Input: part model. Units: mm. Frame: model coordinates. Face numbers are marked on the shaded views. A direction names the side the tool comes from. Coordinates: 2 decimals unless noted, no trailing zeros. Write each loop counter-clockwise with the first axis right and the second up, starting at its lowest first coordinate (ties: lowest second). Pieces come first, ordered by that corner, then holes. Notation, with made-up numbers: (47.5, 44.5) -> (89.5, 44.5) arc R3 ccw to (89.5, 49.5) -> close; hole circle Ø3 at (28.25, -29). An arc over 180 degrees is marked (long way). Use one line per item in the form item = value. Start each with the question number.
(1) Set-up query: the marked faces 1 and 2. Return all of +Z, -Z, +X, -X, +Y, -Y with unobstructed straight access to the full face (end or side cutting, diameter ignored); none if empty.
(2) Pull-direction query (Z, two-part tool) for the marked faces 3, 4, 5 and 6; classes: released by +Z, released by -Z, zero draft, split by the parting line, or undercut.
(3) First-contact query: pin 1 (2.5 mm diameter, centred on x = 12.5, z = 1.5, fed in from +Y); pin 2 (12 mm diameter, centred on x = -7.5, y = 8, fed in from +Z); pin 3 (1.5 mm diameter, centred on x = 13.5, z = 1, fed in from +Y); pin 4 (13 mm diameter, centred on x = -8, y = -6, fed in from -Z). Flat tips, straight axial feed; report the tip coordinate or a pass-through.
(4) Cut plane A-A on x = 12.5. Return the cut outline in (y, z), plus the area to 3 significant figures.
(5) Ray query, line 1 along Y through (x, z) = (13.5, 3.1); line 2 along Y through (x, z) = (-9.5, 2.85); line 3 along X through (y, z) = (-4.5, 1.85). Return the intervals inside material, ascending.
(6) Cut plane B-B on x = -4.75. Return the cut outline in (y, z).
(7) Cut plane C-C on y = 8.75. State how many separate pieces and enclosed holes the cut face has, plus the area to 3 significant figures.
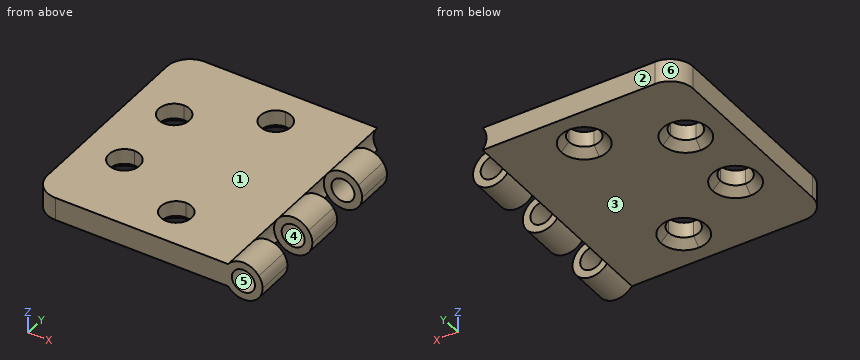
```python
from build123d import *

# Parameters (mm, degrees)
SKETCH_1_W          = 30
SKETCH_1_H          = 30
EXTRUDE_1_DEPTH     = 3
CUT_EXTRUDE_1_DEPTH = 34.674916481
SKETCH_3_R          = 2.5
EXTRUDE_3_DEPTH     = 30
FILLET_1_R          = 3
CUT_EXTRUDE_2_DEPTH = 22.587033145
SKETCH_6_R          = 2.5
CUT_EXTRUDE_3_DEPTH = 5
SKETCH_7_R          = 2.5
CUT_EXTRUDE_4_DEPTH = 5
CUT_EXTRUDE_START   = -5
SKETCH_8_R          = 2.5
CUT_EXTRUDE_5_DEPTH = 5
SKETCH_9_R          = 1.5
CUT_EXTRUDE_6_DEPTH = 34.778691508
CHAMFER_1_SIZE      = 1


with BuildPart() as part:
    # Эскиз1 → Бобышка-Вытянуть1 (new body)
    with BuildSketch(Plane.XY):
        Rectangle(SKETCH_1_W, SKETCH_1_H)
    extrude(amount=EXTRUDE_1_DEPTH)

    # Эскиз2 → Вырез-Вытянуть1 (cut, through all)
    with BuildSketch(Plane.XZ.offset(15)):
        with BuildLine():
            Line((15, 0), (15, 1.5))
            ThreePointArc((15, 1.5), (14.871708245, 0.709430585), (14.5, 0))
            Line((14.5, 0), (15, 0))
        make_face()
        with BuildLine():
            ThreePointArc((14.5, 3), (14.871708245, 2.290569415), (15, 1.5))
            Line((15, 1.5), (15, 3))
            Line((15, 3), (14.5, 3))
        make_face()
    extrude(amount=-CUT_EXTRUDE_1_DEPTH, mode=Mode.SUBTRACT)

    # Эскиз3 → Бобышка-Вытянуть3 (add)
    with BuildSketch(Plane.XZ.offset(15)):
        with Locations((12.5, 1.5)):
            Circle(SKETCH_3_R)
    extrude(amount=-EXTRUDE_3_DEPTH)

    # Скругление1
    fillet_1_edges = [part.edges().sort_by_distance(p)[0] for p in [
        (-15, -15, 1.5),
        (-15, 15, 1.5),
    ]]
    fillet(fillet_1_edges, radius=FILLET_1_R)

    # Эскиз4 → Вырез-Вытянуть2 (cut, through all)
    with BuildSketch(Plane.XY.offset(3)):
        with BuildLine():
            ThreePointArc((-7.5, -5), (-8.085786438, -3.585786438), (-9.5, -3))
            Line((-9.5, -3), (-9.5, -7))
            ThreePointArc((-9.5, -7), (-8.085786438, -6.414213562), (-7.5, -5))
        make_face()
        with BuildLine():
            Line((-9.5, -7), (-9.5, -3))
            ThreePointArc((-9.5, -3), (-11.5, -5), (-9.5, -7))
        make_face()
        with BuildLine():
            ThreePointArc((0.5, -8), (-1.5, -10), (0.5, -12))
            Line((0.5, -12), (0.5, -8))
        make_face()
        with BuildLine():
            Line((0.5, -8), (0.5, -12))
            ThreePointArc((0.5, -12), (1.914213562, -11.414213562), (2.5, -10))
            ThreePointArc((2.5, -10), (1.914213562, -8.585786438), (0.5, -8))
        make_face()
        with BuildLine():
            ThreePointArc((-9.5, 7), (-11.5, 5), (-9.5, 3))
            Line((-9.5, 3), (-9.5, 5))
            Line((-9.5, 5), (-9.5, 7))
        make_face()
        with BuildLine():
            Line((-9.5, 5), (-9.5, 3))
            ThreePointArc((-9.5, 3), (-8.085786438, 3.585786438), (-7.5, 5))
            ThreePointArc((-7.5, 5), (-8.085786438, 6.414213562), (-9.5, 7))
            Line((-9.5, 7), (-9.5, 5))
        make_face()
        with BuildLine():
            ThreePointArc((0.5, 12), (-1.5, 10), (0.5, 8))
            Line((0.5, 8), (0.5, 10))
            Line((0.5, 10), (0.5, 12))
        make_face()
        with BuildLine():
            Line((0.5, 10), (0.5, 8))
            ThreePointArc((0.5, 8), (1.914213562, 8.585786438), (2.5, 10))
            ThreePointArc((2.5, 10), (1.914213562, 11.414213562), (0.5, 12))
            Line((0.5, 12), (0.5, 10))
        make_face()
    extrude(amount=-CUT_EXTRUDE_2_DEPTH, mode=Mode.SUBTRACT)

    # Эскиз6 → Вырез-Вытянуть3 (cut)
    with BuildSketch(Plane(origin=(0, -10, 0), x_dir=(-1, 0, 0), z_dir=(0, -1, 0))):
        with Locations((-12.5, -1.5)):
            Circle(SKETCH_6_R)
    extrude(amount=-CUT_EXTRUDE_3_DEPTH, mode=Mode.SUBTRACT)

    # Эскиз7 → Вырез-Вытянуть4 (cut)
    with BuildSketch(Plane(origin=(0, 0, 0), x_dir=(-1, 0, 0), z_dir=(0, -1, 0))):
        with Locations((-12.5, -1.5)):
            Circle(SKETCH_7_R)
    extrude(amount=-CUT_EXTRUDE_4_DEPTH, mode=Mode.SUBTRACT)

    # Эскиз8 → Вырез-Вытянуть5 (cut)
    with BuildSketch(Plane(origin=(0, 15, 0), x_dir=(1, 0, 0), z_dir=(0, 1, 0)).offset(CUT_EXTRUDE_START)):
        with Locations((12.5, -1.5)):
            Circle(SKETCH_8_R)
    extrude(amount=CUT_EXTRUDE_5_DEPTH, mode=Mode.SUBTRACT)

    # Эскиз9 → Вырез-Вытянуть6 (cut, through all)
    with BuildSketch(Plane.XZ.offset(15)):
        with Locations(Location((12.5, 1.5, 0), (0, 0, 270))):
            Circle(SKETCH_9_R)
    extrude(amount=-CUT_EXTRUDE_6_DEPTH, mode=Mode.SUBTRACT)

    # Фаска1
    chamfer_1_edges = [part.edges().sort_by_distance(p)[0] for p in [
        (-9.5, -3, 0),
        (0.5, -8, 0),
        (-9.5, 3, 0),
        (0.5, 8, 0),
    ]]
    chamfer(chamfer_1_edges, length=CHAMFER_1_SIZE)


solid = part.part
```
Values:
q1.face_1 = +Z, -X, +Y, -Y
q1.face_2 = +Z, -Z, +X, -X, +Y
q2.face_3 = released by -Z
q2.face_4 = undercut
q2.face_5 = undercut
q2.face_6 = zero draft
q3.pin_1 = through
q3.pin_2 = 3
q3.pin_3 = 10
q3.pin_4 = 0
q4.outline = (-15, -1) -> (-10, -1) -> (-10, 0) -> (-15, 0) -> close; (-15, 3) -> (-10, 3) -> (-10, 4) -> (-15, 4) -> close; (-5, -1) -> (0, -1) -> (0, 0) -> (-5, 0) -> close; (-5, 3) -> (0, 3) -> (0, 4) -> (-5, 4) -> close; (5, -1) -> (10, -1) -> (10, 0) -> (5, 0) -> close; (5, 3) -> (10, 3) -> (10, 4) -> (5, 4) -> close
q4.area = 30.0 mm2
q5.line_1 = -15 to -10, -5 to 0, 5 to 10
q5.line_2 = -15 to -7, -3 to 3, 7 to 15
q5.line_3 = -15 to -11.44, -7.56 to 11.04, 13.96 to 14.98
q6.outline = (-15, 0) -> (15, 0) -> (15, 3) -> (-15, 3) -> close
q7.separate_pieces = 2
q7.enclosed_holes = 1
q7.area = 77.5 mm2
